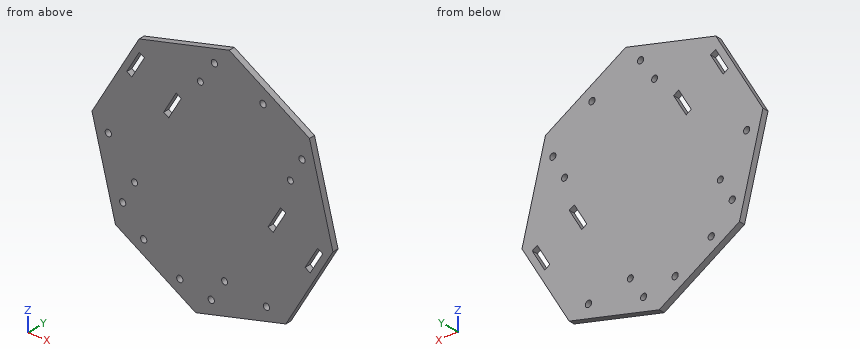
```python
from build123d import *

# Parameters (mm, degrees)
BOSS_EXTRUDE1_DEPTH = 3
SKETCH2_R           = 1.5875
SKETCH2_R_2         = 1.524
CUT_EXTRUDE1_DEPTH  = 3


with BuildPart() as part:
    # Sketch1 → Boss-Extrude1 (new body)
    with BuildSketch(Plane(origin=(-113.226454214, -170.109741769, -309.439751514), x_dir=(0.890793361, 0, -0.454408614), z_dir=(0, -1, 0))):
        Polygon((16.200077076, -64.648683729), (51.592412285, -33.201987218), (54.382400165, 14.060345359), (22.935703655, 49.452680569), (-24.326628923, 52.242668449), (-59.718964132, 20.795971938), (-62.508952012, -26.466360639), (-31.062255502, -61.858695849), align=None)
    extrude(amount=BOSS_EXTRUDE1_DEPTH)

    # Sketch2 → Cut-Extrude1 (cut)
    with BuildSketch(Plane.XZ.offset(173.109741769)):
        with Locations((-172.64368154, -311.255818085)):
            Circle(SKETCH2_R)
        with Locations((-165.337130549, -339.316642084)):
            Circle(SKETCH2_R)
        with Locations((-154.635807236, -351.670528307)):
            Circle(SKETCH2_R)
        with Locations((-159.276542973, -328.182647353)):
            Circle(SKETCH2_R_2)
        with Locations((-125.832608107, -271.190808365)):
            Circle(SKETCH2_R_2)
        with Locations((-118.673164362, -260.366927273)):
            Circle(SKETCH2_R)
        with Locations((-80.052844095, -298.055276559)):
            Circle(SKETCH2_R_2)
        with Locations((-74.095129755, -286.526196957)):
            Circle(SKETCH2_R)
        with Locations((-136.265254, -362.450731171)):
            Circle(SKETCH2_R)
        with Locations((-120.261137836, -365.768123404)):
            Circle(SKETCH2_R)
        with Locations((-113.496778962, -355.047115547)):
            Circle(SKETCH2_R_2)
        with Locations((-92.200313837, -358.461572413)):
            Circle(SKETCH2_R)
        with Locations((-93.954162759, -269.305623721)):
            Circle(SKETCH2_R)
        Polygon((-163.258580453, -280.538613217), (-160.671178566, -282.056951662), (-154.290364989, -271.183401601), (-156.877766876, -269.665063156), align=None)
        Polygon((-144.485366677, -291.620563992), (-141.897964791, -293.138902436), (-135.511480905, -282.255689599), (-138.098882792, -280.737351154), align=None)
        Polygon((-63.58013806, -324.413951361), (-66.167539946, -322.895612916), (-72.548353524, -333.769162977), (-69.960951637, -335.287501422), align=None)
        Polygon((-82.404827782, -313.419720793), (-84.992229669, -311.901382348), (-91.378713554, -322.784595186), (-88.791311667, -324.302933631), align=None)
    extrude(amount=-CUT_EXTRUDE1_DEPTH, mode=Mode.SUBTRACT)


solid = part.part
```
The model under review builds one solid part; all positions refer to its coordinate system, in mm. Coordinates: 2 decimals unless noted, no trailing zeros. Write each loop counter-clockwise with the first axis right and the second up, starting at its lowest first coordinate (ties: lowest second). Pieces come first, ordered by that corner, then holes. Notation, with made-up numbers: (62.5, 46.25) - (72.5, 46.25) arc R15 cw to (72.5, 55.25) - close; hole circle Ø5 at (4.25, 55.5). An arc over 180 degrees is marked (long way). Write item = value, one per line.
(1) For P1, Ø1.9, axis at x = -92.2, z = -358.46, coming from the +Y side; P2, Ø1, axis at y = -171.5, z = -278.5, coming from the +X side; P3, Ø1.5, axis at x = -98.5, y = -172.5, coming from the -Z side; P4, Ø1.5, axis at x = -96.5, y = -172.5, coming from the +Z side, all flat-tipped, find the tip position at first contact; note any pin that passes through.
Result sheet:
P1 = through
P2 = -69.49
P3 = -366.86
P4 = -260.01
(2) Consider section A-A, the plane z = -319. Give the boundary of the cut face in (x, y).
Result sheet:
outline = (-177.19, -173.11) - (-89.16, -173.11) - (-89.16, -170.11) - (-177.19, -170.11) - close; (-85.68, -173.11) - (-59.08, -173.11) - (-59.08, -170.11) - (-85.68, -170.11) - close
(3) For line 1 (X direction, y = -170.9, z = -322.5); line 2 (Z direction, x = -75.5, y = -172.9); line 3 (X direction, y = -172.95, z = -298), list the stretches that pass through material, from the lowest coordinate up. Write a range as [from, to].
Result sheet:
line_1 = [-176.28, -91.21], [-87.73, -58.91]
line_2 = [-350.78, -287.27], [-285.79, -272.77]
line_3 = [-177.06, -81.58], [-78.53, -64.55]
(4) Consider section C-C, the plane x = -97. Give the boundary of the cut face in (y, z), then the cut area to 3 significant figures.
Result sheet:
outline = (-173.11, -366.27) - (-170.11, -366.27) - (-170.11, -260.16) - (-173.11, -260.16) - close
area = 318 mm^2
(5) Consider section D-D, the plane z = -346. Give the boundary of the cut face in (x, y), then the cut area to 3 significant figures.
Result sheet:
outline = (-170.16, -173.11) - (-72.7, -173.11) - (-72.7, -170.11) - (-170.16, -170.11) - close
area = 292 mm^2
(6) Consider section B-B, the plane y = -171.2. State how many separate pieces and enclosed holes the cut face has, then the cut area to 3 significant figures.
Result sheet:
separate_pieces = 1
enclosed_holes = 17
area = 10,600 mm^2
